For this review, take the finished solid that the model builds, in its own axes (mm). Give positions to 0.01 mm unless a question says otherwise; leave off trailing zeros. Write each loop counter-clockwise with the first axis right and the second up, starting at its lowest first coordinate (ties: lowest second). Pieces come first, ordered by that corner, then holes.
1) We need section A-A on y = -148.5. Give the boundary of the cut face in (x, z).
2) We need section B-B on z = -61.5. Give the boundary of the cut face in (x, y).
3) For P1, Ø3, axis at y = -85, z = 255.5, coming from the -X side; P2, Ø3, axis at x = 16.5, z = 0.5, coming from the -Y side; P3, Ø2, axis at y = 186, z = 256, coming from the +X side; P4, Ø3, axis at x = 18.5, y = 60.5, coming from the +Z side, all flat-tipped, find the tip position at first contact; note any pin that passes through.
4) Wall thickness on line 1 along X through (y, z) = (97.5, 308); line 2 along Z through (x, y) = (13, 50): over which ranges is each line inside the solid? List them lowest first.
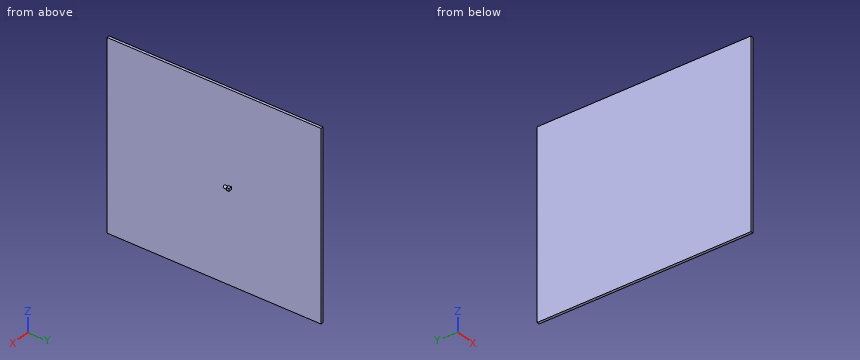
from build123d import *

# Parameters (mm, degrees)
SKETCH1_W           = 711.2
SKETCH1_H           = 812.8
BOSS_EXTRUDE1_DEPTH = 10
SKETCH2_W           = 10
SKETCH2_H           = 10
BOSS_EXTRUDE2_DEPTH = 12.7
SKETCH4_R           = 5.335
BOSS_EXTRUDE5_DEPTH = 12.7


with BuildPart() as part:
    # Sketch1 → Boss-Extrude1 (new body)
    with BuildSketch(Plane(origin=(0, 0, 0), x_dir=(0, 0, -1), z_dir=(1, 0, 0))):
        Rectangle(SKETCH1_W, SKETCH1_H)
    extrude(amount=BOSS_EXTRUDE1_DEPTH)

    # Sketch2 → Boss-Extrude2 (add)
    with BuildSketch(Plane(origin=(10, 0, 0), x_dir=(0, 0, -1), z_dir=(1, 0, 0))):
        with Locations((0, 61.3)):
            Rectangle(SKETCH2_W, SKETCH2_H)
    extrude(amount=BOSS_EXTRUDE2_DEPTH)

    # Sketch4 → Boss-Extrude5 (add)
    with BuildSketch(Plane.XZ.offset(-56.3)):
        with Locations(Location((16, 0, 0), (0, 0, 69.587697496))):
            Circle(SKETCH4_R)
    extrude(amount=BOSS_EXTRUDE5_DEPTH)


solid = part.part
Results list:
1. outline: (0, -355.6) - (10, -355.6) - (10, 355.6) - (0, 355.6) - close
2. outline: (0, -406.4) - (10, -406.4) - (10, 406.4) - (0, 406.4) - close
3. P1: stops at x = 0
3. P2: stops at y = 43.6
3. P3: stops at x = 10
3. P4: stops at z = 5
4. line 1: x = 0 to 10
4. line 2: z = -4.41 to 4.41
